Input: part model. Units: mm. Frame: model coordinates. A direction names the side the tool comes from. Round coordinates to 2 decimals unless told otherwise and drop trailing zeros. Loops run counter-clockwise (first coordinate to the right, second up) from the corner with the lowest first, then second, coordinate; pieces in that order, holes last.
1) First-contact query: pin 1 (4.5 mm diameter, centred on x = -2.5, z = -10.5, fed in from +Y); pin 2 (4.5 mm diameter, centred on x = -1.5, z = -13.5, fed in from -Y); pin 3 (11 mm diameter, centred on x = 0.5, y = 2, fed in from -Z); pin 4 (12 mm diameter, centred on x = 62, y = 5.5, fed in from -Z). Flat tips, straight axial feed; report the tip coordinate or a pass-through.
2) Draft query along X for faces 5 (the face through (-1, -79.5, 4)), 6 (the face through (0, 7, -20)), 7 (the face through (-39, 55.5, 2)). Return one class per face: pulls with the +X half, pulls with the -X half, needs draft (parallel to the pull), parting line crosses it, or undercut.
3) Section D-D, the plane x = -34. Return loops of the section in (y, z).
4) Section C-C, the plane y = 42.5. Return loops of the section in (x, z).
5) Access query for faces 1 (the face through (7.5, 0, -4)), 2 (the face through (-7.5, 0, -4)), 3 (the face through (-1, 1, 5)), 4 (the face through (36, -8.5, 2)). Directions: +Z, -Z, +X, -X, +Y, -Y. A direction counts if a zero-diameter tool reaches every point of the face in a straight line with its end or side. Return the directions, or none.
6) Section A-A, the plane z = -7. Return loops of the section in (x, y), and give its area (3 significant figures).
7) Ray query, line 1 along Y through (x, z) = (51.5, 0.5); line 2 along X through (y, z) = (0.5, 3.5); line 3 along X through (y, z) = (-6.1, -14). Return the intervals inside material, ascending.
8) Section B-B, the plane x = 12. Return loops of the section in (y, z), and give its area (3 significant figures).
from build123d import *

# Parameters (mm, degrees)
SKETCH001_W          = 180
SKETCH001_H          = 159
PAD001_DEPTH         = 8
SKETCH002_W          = 55
SKETCH002_H          = 111
SKETCH002_W_2        = 57
SKETCH002_H_2        = 47
POCKET_DEPTH         = 8.001
SKETCH013_W          = 15
SKETCH013_H          = 20
PAD006_DEPTH         = 20
SKETCH014_W          = 10
SKETCH014_H          = 15
POCKET001_DEPTH      = 90.001
POCKET001_DEPTH_BACK = 90.001
SKETCH015_R          = 1.5
POCKET002_DEPTH      = 79.501
POCKET002_DEPTH_BACK = 79.501
SKETCH016_W          = 165
SKETCH016_H          = 144
POCKET003_DEPTH      = 3


with BuildPart() as part:
    # Sketch001 → Pad001 (new body)
    with BuildSketch(Plane.XY):
        Rectangle(SKETCH001_W, SKETCH001_H)
    extrude(amount=PAD001_DEPTH)

    # Sketch002 → Pocket (cut, through all)
    with BuildSketch(Plane(origin=(0, 0, 0), x_dir=(1, 0, 0), z_dir=(0, 0, -1))):
        with Locations((-38.5, 0)):
            Rectangle(SKETCH002_W, SKETCH002_H)
        with Locations((36.5, 32)):
            Rectangle(SKETCH002_W_2, SKETCH002_H_2)
        with Locations((36.5, -32)):
            Rectangle(SKETCH002_W_2, SKETCH002_H_2)
    extrude(amount=-POCKET_DEPTH, mode=Mode.SUBTRACT)

    # Sketch013 (on DatumPlane) → Pad006 (join)
    with BuildSketch(Plane.XY):
        Rectangle(SKETCH013_W, SKETCH013_H)
    extrude(amount=-PAD006_DEPTH)

    # Sketch014 (on Plane of DatumPlane002) → Pocket001 (cut, two sides)
    with BuildSketch(Plane.YZ) as pocket001_sk:
        with Locations((0, -12.5)):
            Rectangle(SKETCH014_W, SKETCH014_H)
    extrude(amount=-POCKET001_DEPTH, mode=Mode.SUBTRACT)
    extrude(pocket001_sk.sketch, amount=POCKET001_DEPTH_BACK, mode=Mode.SUBTRACT)

    # Sketch015 (on DatumPlane) → Pocket002 (cut, two sides)
    with BuildSketch(Plane.XZ) as pocket002_sk:
        with Locations((0, -14)):
            Circle(SKETCH015_R)
        with BuildLine():
            ThreePointArc((-7.5, -15.941091), (0, -20), (7.5, -15.941091))
            Line((7.5, -15.941091), (9.5, -15.941091))
            Line((9.5, -15.941091), (9.5, -32.907985))
            Line((9.5, -32.907985), (-9.5, -32.907985))
            Line((-9.5, -32.907985), (-9.5, -15.941091))
            Line((-9.5, -15.941091), (-7.5, -15.941091))
        make_face()
    extrude(amount=-POCKET002_DEPTH, mode=Mode.SUBTRACT)
    extrude(pocket002_sk.sketch, amount=POCKET002_DEPTH_BACK, mode=Mode.SUBTRACT)

    # Sketch016 (on DatumPlane) → Pocket003 (cut)
    with BuildSketch(Plane.XY.offset(8)):
        Rectangle(SKETCH016_W, SKETCH016_H)
    extrude(amount=-POCKET003_DEPTH, mode=Mode.SUBTRACT)


solid = part.part
Final values:
1. pin 1: stops at y = 10
1. pin 2: stops at y = -10
1. pin 3: stops at z = -20
1. pin 4: stops at z = 0
2. face 5: needs draft
2. face 6: parting line crosses it
2. face 7: undercut
3. outline: (-79.5, 0) - (-55.5, 0) - (-55.5, 5) - (-72, 5) - (-72, 8) - (-79.5, 8) - close; (55.5, 0) - (79.5, 0) - (79.5, 8) - (72, 8) - (72, 5) - (55.5, 5) - close
4. outline: (-90, 0) - (-66, 0) - (-66, 5) - (-82.5, 5) - (-82.5, 8) - (-90, 8) - close; (-11, 0) - (8, 0) - (8, 5) - (-11, 5) - close; (65, 0) - (90, 0) - (90, 8) - (82.5, 8) - (82.5, 5) - (65, 5) - close
5. face 1: -Z, +X, +Y, -Y
5. face 2: -Z, -X, +Y, -Y
5. face 3: +Z
5. face 4: +Z, -Z
6. outline: (-7.5, -10) - (7.5, -10) - (7.5, -5) - (-7.5, -5) - close; (-7.5, 5) - (7.5, 5) - (7.5, 10) - (-7.5, 10) - close
6. area: 150 mm2
7. line 1: y = -79.5 to -55.5, -8.5 to 8.5, 55.5 to 79.5
7. line 2: x = -90 to -66, -11 to 90
7. line 3: x = -7.5 to -1.5, 1.5 to 7.5
8. outline: (-79.5, 0) - (-55.5, 0) - (-55.5, 5) - (-72, 5) - (-72, 8) - (-79.5, 8) - close; (-8.5, 0) - (8.5, 0) - (8.5, 5) - (-8.5, 5) - close; (55.5, 0) - (79.5, 0) - (79.5, 8) - (72, 8) - (72, 5) - (55.5, 5) - close
8. area: 370 mm2
